The model under review builds one solid part; all positions refer to its coordinate system, in mm. A direction names the side the tool comes from. Round coordinates to 2 decimals unless told otherwise and drop trailing zeros. Order: outer loops, then holes, each group sorted by start corner. A loop starts at its lowest first (then second) coordinate and runs counter-clockwise, first axis right, second up. Notation, with made-up numbers: (41, -13) -> (49, -13) arc R24 ccw to (49, 5) -> close; hole circle Ø11 at (43, 39.25). An arc over 180 degrees is marked (long way). Use a Markdown table: item, result. Add a question column.
```python
from build123d import *

# Parameters (mm, degrees)
SKETCH_2_R          = 7.5
CUT_EXTRUDE_1_DEPTH = 53.668776329


with BuildPart() as part:
    # Эскиз1 → Повернуть4 (revolve)
    with BuildSketch(Plane.XY, mode=Mode.PRIVATE) as revolve_4_sk:
        Polygon((5.5, 35), (7.5, 35), (7.5, 32), (9, 29), (9, 26.999352312), (7.5, 24), (7.5, 0), (-7.5, 0), (-7.5, 24), (-9, 26.999352312), (-9, 29), (-7.5, 32), (-7.5, 35), (-5.5, 35), (-1.75, 18), (1.75, 18), align=None)
    revolve(revolve_4_sk.sketch.rotate(Axis((0, 0, 0), (1, 0, 0)), 180), axis=Axis((0, 0, 0), (1, 0, 0)))

    # Эскиз2 → Вырез-Вытянуть1 (cut, through all)
    with BuildSketch(Plane(origin=(9, 0, 0), x_dir=(0, 0, -1), z_dir=(1, 0, 0))):
        with Locations(Location((0, 0, 0), (0, 0, 90))):
            Circle(SKETCH_2_R)
    extrude(amount=-CUT_EXTRUDE_1_DEPTH, mode=Mode.SUBTRACT)


solid = part.part
```
Q1. Machinability: for faces 1 (the flat face through (7.5, -15.4, 28.4)), 2 (the conical face through (-7.594, -11.161, 21.459)), 3 (the cylindrical face through (0.024, 13.267, -12.165)), which of the approach directions +Z, -Z, +X, -X, +Y, -Y give a long, thin tool a straight path to every point of the face, cutting with its end or side? Answer none if there is none.
Q2. Insertion check: pin 1 (14.5 mm diameter, centred on y = 0.5, z = -1.5, fed in from -X); pin 2 (4 mm diameter, centred on x = -4.5, z = -22, fed in from +Y); pin 3 (24 mm diameter, centred on y = -12, z = -6.5, fed in from +X); pin 4 (10 mm diameter, centred on y = -14.5, z = -22.5, fed in from +X). Each pin has a flat end and moves straight along its axis. Give the tip position at first contact, or say it passes through.
Q3. Wall thickness on line 1 (X direction, y = 9, z = 21.5); line 2 (Y direction, x = -1.25, z = -3.5); line 3 (Z direction, x = -1.5, y = 0): over which ranges is each line inside the solid? List them lowest first. Write a range as [from, to].
Q4. Add section C-C (x = -0.75). Write out the cut boundary in (y, z), then the cut area to 3 significant figures.
Q5. Mouldability with a two-part tool opening along Z and no side actions: class faces 4 (the conical face through (1.985, -18.183, -5.726)), 5 (the flat face through (-7.5, 5, -6)), 6 (the conical face through (7.573, 3.143, -23.94)), 7 (the flat face through (-7.5, 15.4, 28.4)) as pulls with the +Z half, pulls with the -Z half, needs draft (parallel to the pull), parting line crosses it, or undercut.
Report:
| question | item | result |
|---|---|---|
| 1 | face 1 | +X |
| 1 | face 2 | -X |
| 1 | face 3 | none |
| 2 | pin 1 | stops at x = -7.5 |
| 2 | pin 2 | stops at y = 28.53 |
| 2 | pin 3 | stops at x = 8.32 |
| 2 | pin 4 | stops at x = 9 |
| 3 | line 1 | x = [-7.5, -2.92], [2.92, 7.5] |
| 3 | line 2 | y = [-17.66, -6.63], [6.63, 17.66] |
| 3 | line 3 | z = [-18, -7.5], [7.5, 18] |
| 4 | outline | circle Ø36 at (0, 0); hole circle Ø15 at (0, 0) |
| 4 | area | 841 mm² |
| 5 | face 4 | parting line crosses it |
| 5 | face 5 | undercut |
| 5 | face 6 | undercut |
| 5 | face 7 | needs draft |
